```python
from build123d import *

# Parameters (mm, degrees)
F0_W           = 375
F0_H           = 165
F1_DEPTH       = 22
F2_W           = 375
F2_H           = 95
F3_DEPTH       = 95
F4_R           = 10
F6_DEPTH       = 87.5
F7_W           = 6
F7_H           = 110
F8_DEPTH       = 77.5
F9_R           = 30
F10_R          = 51
F10_R_2        = 31
F10_R_3        = 18
F11_DEPTH      = 87.501
F11_DEPTH_BACK = 87.501
F12_W          = 366
F12_H          = 75
F13_DEPTH      = 120
F14_R          = 10
F15_DEPTH      = 25


with BuildPart() as f1:
    # F0 (on Top) → F1 (new body)
    with BuildSketch(Plane.XY):
        Rectangle(F0_W, F0_H)
    extrude(amount=F1_DEPTH)

    # F2 (on face) → F3 (join)
    with BuildSketch(Plane.XY.offset(22)):
        Rectangle(F2_W, F2_H)
    extrude(amount=F3_DEPTH)

    # F4
    f4_edges = [f1.edges().sort_by_distance(p)[0] for p in [
        (-187.5, -82.5, 11),
        (187.5, -82.5, 11),
        (187.5, 82.5, 11),
        (187.5, 47.5, 69.5),
        (187.5, -47.5, 69.5),
        (-187.5, -47.5, 69.5),
        (-187.5, 47.5, 69.5),
        (-187.5, 82.5, 11),
    ]]
    fillet(f4_edges, radius=F4_R)

    # F5 (on Front) → F6 (join, symmetric)
    with BuildSketch(Plane.XZ):
        with BuildLine():
            Line((223, 132), (-223, 132))
            Line((-223, 132), (-223, 117))
            Line((-223, 117), (-157.864934582, 117))
            Line((-157.864934582, 117), (-157.864934582, 99))
            Line((-157.864934582, 99), (-125.864934582, 99))
            ThreePointArc((-125.864934582, 99), (-63, 61), (-0.135065418, 99))
            Line((-0.135065418, 99), (29.9531592821, 99))
            ThreePointArc((29.9531592821, 99), (62, 86), (94.0468407179, 99))
            Line((94.0468407179, 99), (142, 99))
            ThreePointArc((142, 99), (159.2336879396, 103.8575054411), (171.3938769134, 117))
            Line((171.3938769134, 117), (223, 117))
            Line((223, 117), (223, 132))
        make_face()
    extrude(amount=F6_DEPTH, both=True)

    # F7 (on Front) → F8 (join, symmetric)
    with BuildSketch(Plane.XZ):
        with Locations((-63, 77)):
            Rectangle(F7_W, F7_H)
        with Locations((62, 77)):
            Rectangle(F7_W, F7_H)
        with Locations((142, 77)):
            Rectangle(F7_W, F7_H)
        Polygon((-44.7298753819, 77.0821119323), (-11.1961524227, 19), (-6, 22), (-39.5337229592, 80.0821119323), align=None)
        Polygon((-86.4662770408, 80.0821119323), (-120, 22), (-114.8038475773, 19), (-81.2701246181, 77.0821119323), align=None)
    extrude(amount=F8_DEPTH, both=True)

    # F9
    f9_edges = [f1.edges().sort_by_distance(p)[0] for p in [
        (223, -87.5, 124.5),
        (223, 87.5, 124.5),
        (-223, 87.5, 124.5),
        (-223, -87.5, 124.5),
    ]]
    fillet(f9_edges, radius=F9_R)

    # F10 (on Front) → F11 (cut, two sides)
    with BuildSketch(Plane.XZ) as f11_sk:
        with Locations((-63, 132)):
            Circle(F10_R)
        with Locations((62, 132)):
            Circle(F10_R_2)
        with Locations((142, 132)):
            Circle(F10_R_3)
    extrude(amount=-F11_DEPTH, mode=Mode.SUBTRACT)
    extrude(f11_sk.sketch, amount=F11_DEPTH_BACK, mode=Mode.SUBTRACT)

    # F12 (on face) → F13 (cut)
    with BuildSketch(Plane.XY.offset(132)):
        Rectangle(F12_W, F12_H)
    extrude(amount=-F13_DEPTH, mode=Mode.SUBTRACT)

    # F14 (on face) → F15 (cut)
    with BuildSketch(Plane(origin=(0, 0, 0), x_dir=(1, 0, 0), z_dir=(0, 0, -1))):
        with Locations((-167.5, 62.5)):
            Circle(F14_R)
        with Locations((-167.5, -62.5)):
            Circle(F14_R)
        with Locations((167.5, -62.5)):
            Circle(F14_R)
        with Locations((167.5, 62.5)):
            Circle(F14_R)
    extrude(amount=-F15_DEPTH, mode=Mode.SUBTRACT)


solid = f1.part
```
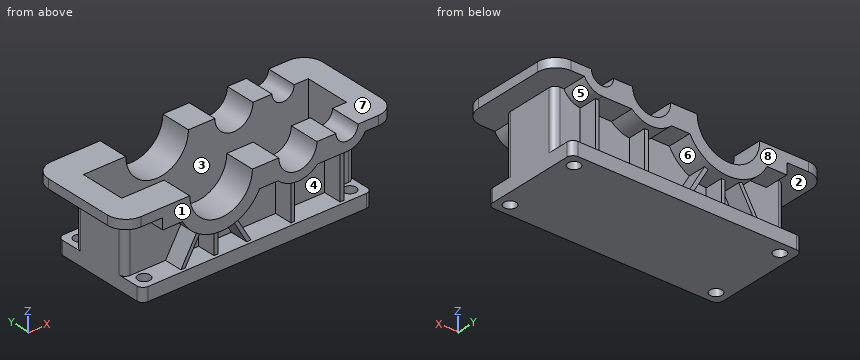
Geometry: final body of the model. Coordinates: model frame, mm. Face numbers are marked on the shaded views. A direction names the side the tool comes from. Give positions to 0.01 mm unless a question says otherwise; leave off trailing zeros. Write each loop counter-clockwise with the first axis right and the second up, starting at its lowest first coordinate (ties: lowest second). Pieces come first, ordered by that corner, then holes.
1. Line query: probe 1 along X at (y, z) = (-62, 13); probe 2 along Y at (x, z) = (-167, 10); probe 3 along Y at (x, z) = (-95.5, 53.5). Output: solid intervals per line, ascending.
2. Draft query along Y for the marked faces 1, 2 and 3. Return one class per face: released by +Y, released by -Y, zero draft, split by the parting line, or undercut.
3. Section query C-C, the plane x = -28. Return loops of the section in (y, z).
4. Section query B-B, the plane y = 23.5. Return loops of the section in (x, z), then the cut area to 4 significant figures.
5. Reachability of the marked faces 4, 5, 6, 7 and 8 from +Z, -Z, +X, -X, +Y, -Y: full face, straight path, thin tool, end or side. Return the list, or none.
6. Section query D-D, the plane y = -62.5. Count the separate pieces of the cut face and the enclosed holes in it, then the cut area to 3 significant figures.
7. Section query A-A, the plane x = -167.5. Return loops of the section in (y, z).
8. Pin query (flat end, axial travel): P1, Ø1.5, axis at x = -166.5, z = 67, coming from the +Y side; P2, Ø1, axis at y = 67, z = 101, coming from the -X side; P3, Ø22.5, axis at y = 12, z = 100, coming from the -X side. Return the tip coordinate at first contact, or that it passes through.
Computed:
1. probe 1: x = -187.5 to -177.49, -157.51 to 157.51, 177.49 to 187.5
1. probe 2: y = -82.5 to -72.49, -52.51 to 52.51, 72.49 to 82.5
1. probe 3: y = -77.5 to -37.5, 37.5 to 77.5
2. face 1: released by -Y
2. face 2: zero draft
2. face 3: undercut
3. outline: (-87.5, 70.23) - (-47.5, 70.23) - (-47.5, 60.11) - (-77.5, 60.11) - (-77.5, 48.11) - (-47.5, 48.11) - (-47.5, 22) - (-82.5, 22) - (-82.5, 0) - (82.5, 0) - (82.5, 22) - (47.5, 22) - (47.5, 48.11) - (77.5, 48.11) - (77.5, 60.11) - (47.5, 60.11) - (47.5, 70.23) - (87.5, 70.23) - (87.5, 94.91) - (37.5, 94.91) - (37.5, 12) - (-37.5, 12) - (-37.5, 94.91) - (-87.5, 94.91) - close
4. outline: (-223, 117) - (-187.5, 117) - (-187.5, 0) - (187.5, 0) - (187.5, 117) - (223, 117) - (223, 132) - (183, 132) - (183, 12) - (-183, 12) - (-183, 132) - (-223, 132) - close
4. area: 6,645 mm2
5. face 4: -Y
5. face 5: +X, +Y
5. face 6: +Y
5. face 7: +Z, +X, -X, +Y, -Y
5. face 8: +Z, -Z, +X, -X, +Y
6. separate pieces: 3
6. enclosed holes: 4
6. area: 19,400 mm2
7. outline: (-87.5, 117) - (-47.5, 117) - (-47.5, 22) - (-52.5, 22) - (-52.5, 0) - (52.5, 0) - (52.5, 22) - (47.5, 22) - (47.5, 117) - (87.5, 117) - (87.5, 132) - (37.5, 132) - (37.5, 12) - (-37.5, 12) - (-37.5, 132) - (-87.5, 132) - close; (-82.5, 0) - (-72.5, 0) - (-72.5, 22) - (-82.5, 22) - close; (72.5, 0) - (82.5, 0) - (82.5, 22) - (72.5, 22) - close
8. P1: stops at y = 47.5
8. P2: stops at x = -157.86
8. P3: stops at x = -187.5
